```python
from build123d import *

# Parameters (mm, degrees)
SALIENTE_EXTRUIR1_DEPTH = 92
CROQUIS3_W              = 3
CROQUIS3_H              = 17
SALIENTE_EXTRUIR2_DEPTH = 3


with BuildPart() as part:
    # Croquis1 → Saliente-Extruir1 (new body)
    with BuildSketch(Plane.XY):
        Polygon((0, 0), (16.069690242, -19.151111078), (13.771556913, -21.079473907), (-2.298133329, -1.928362829), align=None)
    extrude(amount=SALIENTE_EXTRUIR1_DEPTH)

    # Croquis3 → Saliente-Extruir2 (add)
    with BuildSketch(Plane(origin=(-2.298133329, -1.928362829, 0), x_dir=(0, 0, 1), z_dir=(-0.7660444431189819, -0.6427876096865347, 0))):
        with Locations((93.5, -8.5)):
            Rectangle(CROQUIS3_W, CROQUIS3_H)
        with Locations((-1.5, -8.5)):
            Rectangle(CROQUIS3_W, CROQUIS3_H)
    extrude(amount=-SALIENTE_EXTRUIR2_DEPTH)


solid = part.part
```
Work out the finished part from the listing and answer in its coordinate system (mm). A direction names the side the tool comes from. Give positions to 0.01 mm unless a question says otherwise; leave off trailing zeros. Write each loop counter-clockwise with the first axis right and the second up, starting at its lowest first coordinate (ties: lowest second). Pieces come first, ordered by that corner, then holes. Notation, with made-up numbers: (46, -39) -> (99, -39) arc R19 ccw to (99, -23) -> close; hole circle Ø4 at (-18.75, 15.25). An arc over 180 degrees is marked (long way). Write each question's results on one line, items separated by ' | '.
1. Each of these flat-tipped pins is pushed along its axis until it touches: pin 1 Ø8 at (y, z) = (-11.5, 14) entering from +X; pin 2 Ø3 at (x, y) = (10.5, -9) entering from -Z; pin 3 Ø6 at (x, y) = (13.5, -15) entering from +Z; pin 4 Ø5 at (y, z) = (-17.5, 15) entering from -X. Where does it stop, or does it pass through?
Data:
pin 1: x = 13.01 | pin 2: through | pin 3: z = 92 | pin 4: x = 8.67
2. Find section A-A on y = -14. Determine the outline of the cut face in (x, z), and give its area (3 significant figures).
Data:
outline: (7.83, -3) -> (9.76, -3) -> (9.76, 0) -> (11.75, 0) -> (11.75, 92) -> (9.76, 92) -> (9.76, 95) -> (7.83, 95) -> close | area: 372 mm^2
3. Find section B-B on x = 7.5. Determine the outline of the cut face in (y, z), and give its area (3 significant figures).
Data:
outline: (-13.61, -3) -> (-8.94, -3) -> (-8.94, 95) -> (-13.61, 95) -> close | area: 457 mm^2
4. Find section D-D on y = -3.75. Determine the outline of the cut face in (x, z), and give its area (3 significant figures).
Data:
outline: (-0.77, -3) -> (3.15, -3) -> (3.15, 95) -> (-0.77, 95) -> close | area: 384 mm^2
5. Find section C-C on z = 73. Determine the outline of the cut face in (x, y).
Data:
outline: (-2.3, -1.93) -> (13.77, -21.08) -> (16.07, -19.15) -> (0, 0) -> close
6. Straight lines are drawn through the part: L1, parallel to X at y = -2.75, z = 33.5; L2, parallel to Y at x = 14, z = 76; L3, parallel to X at y = -10.5, z = 26. For each, find the intervals that lie inside material, in ascending order.
Data:
L1: -1.61 to 2.31 | L2: -20.89 to -16.68 | L3: 4.89 to 8.81
7. A tool of negligible diameter and unlimited length cuts with its end or side. For faces 1 (the flat face through (9.76, -14, 93.48)), 2 (the flat face through (9.76, -14, -1.52)), 3 (the flat face through (14.94, -20.1, 45.36)), from which of +Z, -Z, +X, -X, +Y, -Y can it reach the whole face along a straight path? Write none if from no direction.
Data:
face 1: +Z, +X, -Y | face 2: -Z, +X, -Y | face 3: +Z, -Z, +X, -Y
